```python
from build123d import *

# Parameters (mm, degrees)
F1_DEPTH = 12.7
F3_DEPTH = 3.175
F4_R     = 2.032
F5_DEPTH = 12.701


with BuildPart() as f1:
    # F0 (on Front) → F1 (new body)
    with BuildSketch(Plane.XZ):
        Polygon((0, 13.4703841816), (0, 17.9605122421), (-17.9605122421, 0), (-13.4703841816, 0), align=None)
    extrude(amount=F1_DEPTH)

    # F2 (on face) → F3 (join)
    with BuildSketch(Plane.XZ.offset(12.7)):
        Polygon((0, 0), (0, 13.4703841816), (-13.4703841816, 0), align=None)
    extrude(amount=-F3_DEPTH)

    # F4 (on face) → F5 (cut, through all)
    with BuildSketch(Plane(origin=(-8.9802561211, 0, 8.9802561211), x_dir=(0, -1, 0), z_dir=(-0.7071067812, 0, 0.7071067812))):
        Circle(F4_R)
    extrude(amount=-F5_DEPTH, mode=Mode.SUBTRACT)

    # F6: F1 across face


with BuildPart() as f1_1:
    add(f1.part)
    add(f1.part.mirror(Plane(origin=(0, -8.3910714286, 11.8667670171), x_dir=(0, 1, 0), z_dir=(1, 0, 0))))

    # F7: F1 across face


with BuildPart() as f1_2:
    add(f1_1.part)
    add(f1_1.part.mirror(Plane(origin=(0, 0, 12.6031300765), x_dir=(-1, 0, 0), z_dir=(0, 1, 0))))


solid = f1_2.part
```
Source: CAD feature listing. Evaluate the final solid. Frame: model axes, mm. A direction names the side the tool comes from. Round coordinates to 2 decimals unless told otherwise and drop trailing zeros. Loops run counter-clockwise (first coordinate to the right, second up) from the corner with the lowest first, then second, coordinate; pieces in that order, holes last.
1. Section query D-D on x = 1. Output: boundary loops of the cut face in (y, z) (3 decimals).
2. Contact query for flat-ended pins moving along their axis: pin 1 (10 mm diameter, centred on x = 5.5, y = -2.5, fed in from +Z); pin 2 (12 mm diameter, centred on x = 5.5, y = -2.5, fed in from -Z); pin 3 (2 mm diameter, centred on y = -9, z = 5, fed in from -X). Output: stop coordinate, or through.
3. Mould query, pull axis X, two halves, no side actions, for faces 3 (the flat face through (-6.86, -0.18, 11.1)), 4 (the flat face through (0, -9.525, 5)), 5 (the flat face through (0, -11, 0)). Classes: released by +X, released by -X, zero draft, split by the parting line, or undercut.
4. Ray query, L1, parallel to Y at x = 3, z = 2 (3 decimals); L2, parallel to X at y = -3.5, z = 5.75; L3, parallel to X at y = 2.75, z = 2. Return the intervals inside material, ascending.
5. Access query for faces 1 (the flat face through (0, 9.525, 5)), 2 (the flat face through (0, 12.7, 7)). Directions: +Z, -Z, +X, -X, +Y, -Y. A direction counts if a zero-diameter tool reaches every point of the face in a straight line with its end or side. Return the directions, or none.
6. Section query C-C on y = -2.75. Output: boundary loops of the cut face in (x, z), and give its area (3 significant figures).
7. Section query A-A on y = 0.5. Output: boundary loops of the cut face in (x, z), and give its area (3 significant figures).
8. Section query B-B on z = 2. Output: boundary loops of the cut face in (x, y) (3 decimals).
Answers below:
1. outline: (-12.7, 0) - (-9.525, 0) - (-9.525, 12.47) - (9.525, 12.47) - (9.525, 0) - (12.7, 0) - (12.7, 16.961) - (-12.7, 16.961) - close
2. pin 1: stops at z = 17.46
2. pin 2: stops at z = 1.97
2. pin 3: stops at x = -13.96
3. face 3: released by -X
3. face 4: undercut
3. face 5: zero draft
4. L1: y = -12.7 to -9.525, 9.525 to 12.7
4. L2: x = -12.21 to -7.72, 7.72 to 12.21
4. L3: x = -15.96 to -11.47, 11.47 to 15.96
5. face 1: -Z
5. face 2: +Z, -Z, +X, -X, +Y
6. outline: (-17.96, 0) - (-13.47, 0) - (0, 13.47) - (13.47, 0) - (17.96, 0) - (0, 17.96) - close
6. area: 141 mm2
7. outline: (-17.96, 0) - (-13.47, 0) - (-8.13, 5.34) - (-10.37, 7.59) - close; (-7.59, 10.37) - (-5.34, 8.13) - (0, 13.47) - (5.34, 8.13) - (7.59, 10.37) - (0, 17.96) - close; (8.13, 5.34) - (13.47, 0) - (17.96, 0) - (10.37, 7.59) - close
7. area: 116 mm2
8. outline: (-15.961, -12.7) - (15.961, -12.7) - (15.961, 12.7) - (-15.961, 12.7) - close; hole (-11.47, -9.525) - (11.47, -9.525) - (11.47, 9.525) - (-11.47, 9.525) - close
